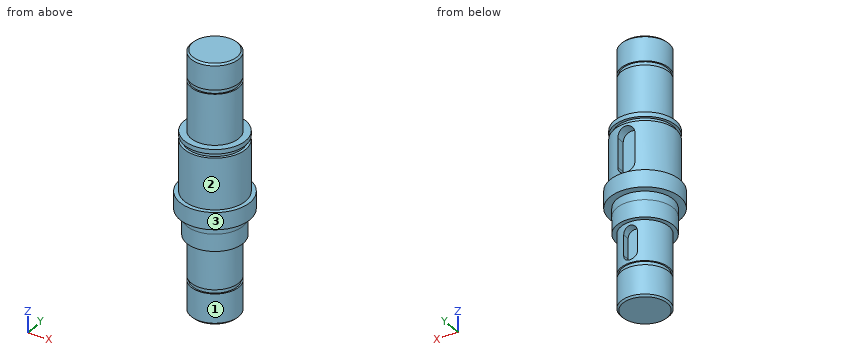
from build123d import *

# Parameters (mm, degrees)
BOSS_EXTRUDE1_DEPTH      = 5
BOSS_EXTRUDE1_DEPTH_BACK = 40
SKETCH1_R                = 18
SKETCH2_R                = 14
BOSS_EXTRUDE2_DEPTH      = 45
SKETCH3_R                = 14
BOSS_EXTRUDE3_DEPTH      = 15
BOSS_EXTRUDE4_START      = 47
SKETCH4_R                = 14
BOSS_EXTRUDE4_DEPTH      = 47
CUT_EXTRUDE1_START       = 1
CUT_EXTRUDE1_DEPTH       = 8
CUT_EXTRUDE2_DEPTH       = 8
SKETCH7_W                = 5.778552493
SKETCH7_H                = 10
SKETCH8_W                = 8.791380579
SKETCH8_H                = 2.4
CUT_EXTRUDE3_START       = -5
SKETCH12_R               = 15.75679301
SKETCH12_R_2             = 13.15
CUT_EXTRUDE3_DEPTH       = 2.4
BOSS_EXTRUDE5_START      = 25
SKETCH11_R               = 16.5
SKETCH11_R_2             = 14
BOSS_EXTRUDE5_DEPTH      = 10
SKETCH15_W               = 6.233882618
SKETCH15_H               = 2.4
CHAMFER1_SIZE            = 1
SKETCH16_R               = 16.5
BOSS_EXTRUDE6_DEPTH      = 10


with BuildPart() as part:
    # Sketch1 → Boss-Extrude1 (new, two sides: drawn at the far end of the back side and taken through both)
    with BuildSketch(Plane.XY.offset(-BOSS_EXTRUDE1_DEPTH_BACK)):
        Circle(SKETCH1_R)
    extrude(amount=BOSS_EXTRUDE1_DEPTH + BOSS_EXTRUDE1_DEPTH_BACK)

    # Sketch2 → Boss-Extrude2 (add)
    with BuildSketch(Plane(origin=(0, 0, -40), x_dir=(-1, 0, 0), z_dir=(0, 0, -1))):
        with Locations(Location((0, 0, 0), (0, 0, 180))):
            Circle(SKETCH2_R)
    extrude(amount=BOSS_EXTRUDE2_DEPTH)

    # Sketch3 → Boss-Extrude3 (add)
    with BuildSketch(Plane(origin=(0, 0, -85), x_dir=(-1, 0, 0), z_dir=(0, 0, -1))):
        with Locations(Location((0, 0, 0), (0, 0, 180))):
            Circle(SKETCH3_R)
    extrude(amount=BOSS_EXTRUDE3_DEPTH)

    # Sketch4 → Boss-Extrude4 (add)
    with BuildSketch(Plane.XY.offset(5).offset(BOSS_EXTRUDE4_START)):
        Circle(SKETCH4_R)
    extrude(amount=-BOSS_EXTRUDE4_DEPTH)

    # Sketch5 → Cut-Extrude1 (cut)
    with BuildSketch(Plane.XZ.offset(-21.3).offset(CUT_EXTRUDE1_START)):
        with BuildLine():
            Line((-5, -6.5), (-5, -23.5))
            ThreePointArc((-5, -23.5), (0, -28.5), (5, -23.5))
            Line((5, -23.5), (5, -6.5))
            ThreePointArc((5, -6.5), (0, -1.5), (-5, -6.5))
        make_face()
    extrude(amount=CUT_EXTRUDE1_DEPTH, mode=Mode.SUBTRACT)

    # Sketch6 → Cut-Extrude2 (cut)
    with BuildSketch(Plane.XZ.offset(-17.3)):
        with BuildLine():
            Line((-4, -61), (-4, -73))
            ThreePointArc((-4, -73), (0, -77), (4, -73))
            Line((4, -73), (4, -61))
            ThreePointArc((4, -61), (0, -57), (-4, -61))
        make_face()
    extrude(amount=CUT_EXTRUDE2_DEPTH, mode=Mode.SUBTRACT)

    # Sketch7 → Revolve1 (revolve)
    with BuildSketch(Plane(origin=(0, 0, 0), x_dir=(1, 0, 0), z_dir=(0, 1, 0))):
        with Locations((17.610723754, 35)):
            Rectangle(SKETCH7_W, SKETCH7_H)
    revolve(axis=Axis((0, 0, -30.114461013), (0, 0, -1)))

    # Sketch8 → Cut-Revolve1 (revolve, cut)
    with BuildSketch(Plane(origin=(0, 0, 0), x_dir=(1, 0, 0), z_dir=(0, 1, 0)), mode=Mode.PRIVATE) as cut_revolve1_sk:
        with Locations((20.79569029, -1.2)):
            Rectangle(SKETCH8_W, SKETCH8_H)
    revolve(cut_revolve1_sk.sketch.rotate(Axis((0, 0, 0), (0, 0, 1)), 180), axis=Axis((0, 0, 0), (0, 0, 1)), mode=Mode.SUBTRACT)

    # Sketch12 → Cut-Extrude3 (cut)
    with BuildSketch(Plane(origin=(0, 0, -83.741663421), x_dir=(-1, 0, 0), z_dir=(0, 0, -1)).offset(CUT_EXTRUDE3_START)):
        Circle(SKETCH12_R)
        Circle(SKETCH12_R_2, mode=Mode.SUBTRACT)
    extrude(amount=CUT_EXTRUDE3_DEPTH, mode=Mode.SUBTRACT)

    # Sketch11 → Boss-Extrude5 (add)
    with BuildSketch(Plane.XY.offset(-60).offset(BOSS_EXTRUDE5_START)):
        Circle(SKETCH11_R)
        Circle(SKETCH11_R_2, mode=Mode.SUBTRACT)
    extrude(amount=-BOSS_EXTRUDE5_DEPTH)

    # Sketch15 → Cut-Revolve2 (revolve, cut)
    with BuildSketch(Plane(origin=(0, 0, 0), x_dir=(1, 0, 0), z_dir=(0, 1, 0)), mode=Mode.PRIVATE) as cut_revolve2_sk:
        with Locations((16.266941309, -35.8)):
            Rectangle(SKETCH15_W, SKETCH15_H)
    revolve(cut_revolve2_sk.sketch.rotate(Axis((0, 0, 52), (0, 0, -1)), 180), axis=Axis((0, 0, 52), (0, 0, -1)), mode=Mode.SUBTRACT)

    # SurfaceCut1
    split(bisect_by=Plane.XY.offset(-99.141663421), keep=Keep.TOP)

    # Chamfer1
    chamfer1_edges = [part.edges().sort_by_distance(p)[0] for p in [
        (-14, 0, 52),
        (-14, 0, -99.141663421),
    ]]
    chamfer(chamfer1_edges, length=CHAMFER1_SIZE)

    # Sketch16 → Boss-Extrude6 (add)
    with BuildSketch(Plane(origin=(0, 0, -45), x_dir=(-1, 0, 0), z_dir=(0, 0, -1))):
        Circle(SKETCH16_R)
    extrude(amount=BOSS_EXTRUDE6_DEPTH)


solid = part.part
Work out the finished part from the listing and answer in its coordinate system (mm). Face numbers are marked on the shaded views. A direction names the side the tool comes from. Give positions to 0.01 mm unless a question says otherwise; leave off trailing zeros. Loops run counter-clockwise (first coordinate to the right, second up) from the corner with the lowest first, then second, coordinate; pieces in that order, holes last. Notation, with made-up numbers: (44, -21) -> (72, -21) arc R17 cw to (72, -8) -> close; hole circle Ø11 at (82.5, -33.5). An arc over 180 degrees is marked (long way). Use a Markdown table: item, result. Add a question column.
1) The part is cut by section C-C, the plane z = 21. Determine the outline of the cut face in (x, y).
2) The part is cut by section B-B, the plane z = -16. Determine the outline of the cut face in (x, y).
3) Each of these flat-tipped pins is pushed along its axis until it touches: P1, Ø1.2, axis at y = 10.5, z = -69, coming from the +X side; P2, Ø1.5, axis at y = 14.5, z = -17.5, coming from the -X side; P3, Ø5, axis at x = 10.5, z = 21.5, coming from the +Y side. Where does it stop, or does it pass through?
4) Which of the six approach directions +Z, -Z, +X, -X, +Y, -Y give full straight-line access (tool end or side, diameter ignored) to the marked faces 1, 2 and 3?
5) Consider line 1 along Z through (x, y) = (-9.5, -15); line 2 along Z through (x, y) = (11.5, 16); line 3 along Y through (x, z) = (1, -51.5). Determine where each line is inside the solid, lowest interval first.
6) The part is cut by section A-A, the plane z = -33. Determine the outline of the cut face in (x, y), plus the area to 3 significant figures.
Reported:
| question | item | result |
|---|---|---|
| 1 | outline | circle Ø28 at (0, 0) |
| 2 | outline | (-5, 12.3) -> (-5, 17.29) arc R18 ccw (long way) to (5, 17.29) -> (5, 12.3) -> close |
| 3 | P1 | stops at x = 9.9 |
| 3 | P2 | stops at x = -11.62 |
| 3 | P3 | stops at y = 11.49 |
| 4 | face 1 | -Z |
| 4 | face 2 | +Z |
| 4 | face 3 | +Z, -Z |
| 5 | line 1 | z = -40 to 0, 2.4 to 5 |
| 5 | line 2 | z = -40 to -30 |
| 5 | line 3 | y = -16.47 to 16.47 |
| 6 | outline | circle Ø41 at (0, 0) |
| 6 | area | 1,320 mm^2 |
